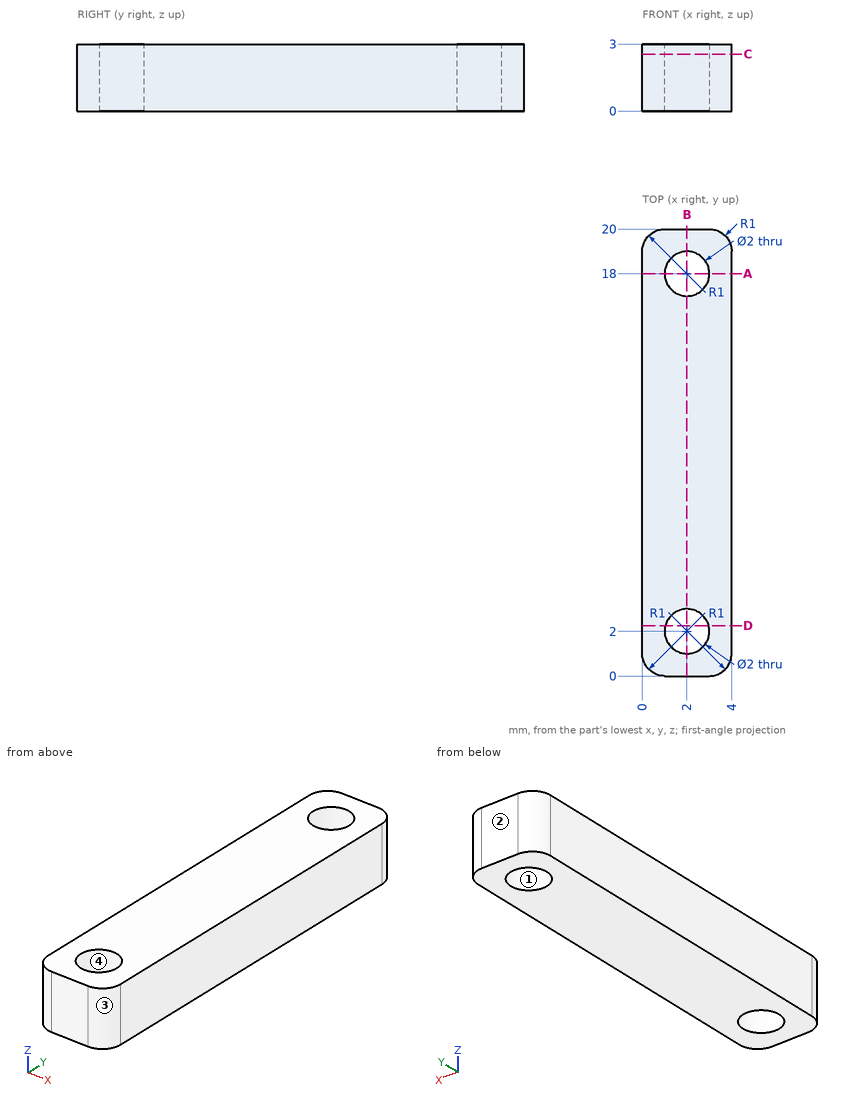
Drawing for the job (mm, zero at the part's lowest x, y, z). Round coordinates to 2 decimals unless told otherwise and drop trailing zeros. Loops run counter-clockwise (first coordinate to the right, second up) from the corner with the lowest first, then second, coordinate; pieces in that order, holes last. Notation, with made-up numbers: (20.5, -29) - (29.5, -29) arc R20 ccw to (29.5, -20) - close; hole circle Ø9 at (-34.75, 51.25). An arc over 180 degrees is marked (long way). Return JSON: item names as keys, results as strings. Group by question number.
Q1. Band-saw the part on C-C on z = 2.55. Give the cut face in (x, y).
Q2. Band-saw the part on D-D on y = 2.25. Give the cut face in (x, z).
Q3. Drill centre lines: line 1 along Y through (x, z) = (2, 1.25); line 2 along Y through (x, z) = (2.75, 0.8); line 3 along X through (y, z) = (18.25, 2). Where is each one in solid material? Low to high. Write a range as [from, to].
Q4. Band-saw the part on A-A on y = 18. Give the cut face in (x, z).
Q5. Band-saw the part on B-B on x = 2. Give the cut face in (y, z), plus the area to 3 significant figures.
Q6. Two-plate mould, pull along X, no slides. Class the marked faces 1, 2, 3 and 4: +X half, -X half, draft (parallel to the pull), parting line (faces both ways), or undercut.
Solutions:
{
 "1": {"outline": "(0, 1) arc R1 ccw to (1, 0) - (3, 0) arc R1 ccw to (4, 1) - (4, 19) arc R1 ccw to (3, 20) - (1, 20) arc R1 ccw to (0, 19) - close; hole circle Ø2 at (2, 2); hole circle Ø2 at (2, 18)"},
 "2": {"outline": "(0, 0) - (1.03, 0) - (1.03, 3) - (0, 3) - close; (2.97, 0) - (4, 0) - (4, 3) - (2.97, 3) - close"},
 "3": {"line 1": "y = [0, 1], [3, 17], [19, 20]", "line 2": "y = [0, 1.34], [2.66, 17.34], [18.66, 20]", "line 3": "x = [0, 1.03], [2.97, 4]"},
 "4": {"outline": "(0, 0) - (1, 0) - (1, 3) - (0, 3) - close; (3, 0) - (4, 0) - (4, 3) - (3, 3) - close"},
 "5": {"outline": "(0, 0) - (1, 0) - (1, 3) - (0, 3) - close; (3, 0) - (17, 0) - (17, 3) - (3, 3) - close; (19, 0) - (20, 0) - (20, 3) - (19, 3) - close", "area": "48.0 mm^2"},
 "6": {"face 1": "undercut", "face 2": "draft", "face 3": "+X half", "face 4": "undercut"}
}
